Can you work these out from the model? Positions are in its coordinate system, mm. Round coordinates to 2 decimals unless told otherwise and drop trailing zeros. Write each question's results on one line, items separated by ' | '.
Autodesk Inventor part; units mm, degrees
ref_plane "YZ Plane" through (0, 0, 0) normal (1, 0, 0) x (0, 1, 0)
ref_plane "XZ Plane" through (0, 0, 0) normal (0, 1, 0) x (-1, 0, 0)
ref_plane "XY Plane" through (0, 0, 0) normal (0, 0, 1) x (1, 0, 0)
sketch "Sketch1" plane through (0, 0, 0) normal (0, 0, 1) x (1, 0, 0)
  line L0 (-90, -105) -> (90, -105)
  line L1 (90, -105) -> (90, 105)
  line L2 (-90, 105) -> (-90, -105)
  line L3 (42, 105) -> (42, 197)
  line L4 (42, 197) -> (-42, 197)
  line L5 (-42, 197) -> (-42, 105)
  line L6 (90, 105) -> (42, 105)
  line L7 (-42, 105) -> (-90, 105)
  point P0 (0, 0)
  dimension "d0" = 180
  dimension "d1" = 210
  dimension "d2" = 105
  dimension "d3" = 90
  dimension "d22" = 92
  dimension "d24" = 42
  dimension "d26" = 84
  dimension "d28" = 92
  dimension "d29" = 210
  dimension "d30" = 48
  dimension "d31" = 48
extrude "Extrusion1" add sketch "Sketch1" along normal blind 2
sketch "Sketch2" plane through (0, 0, 2) normal (0, 0, 1) x (1, 0, 0)
  line L0 (-90, -105) -> (90, -105)
  line L1 (-42, 105) -> (-90, 105)
  point P0 (0, 0)
  point P1 (-75, 80)
  point P2 (75, 80)
  point P3 (-75, -90)
  point P4 (75, -90)
  dimension "d6" = 170
  dimension "d8" = 150
  dimension "d9" = 75
  dimension "d10" = 150
  dimension "d11" = 15
  dimension "d12" = 15
  dimension "d13" = 170
  dimension "d14" = 75
  dimension "d27" = 25
hole "Hole1" at (-75, 80, 2) at (75, 80, 2) at (-75, -90, 2) at (75, -90, 2) direction (0, 0, -1) diameter 4.2 end through all
sketch "Sketch3" plane through (0, 0, 2) normal (0, 0, 1) x (1, 0, 0)
  line L0 (-90, 105) -> (-90, -105)
  line L1 (90, 105) -> (42, 105)
  line L2 (-39, 116) -> (39, 116)
  line L3 (39, 116) -> (39, 194)
  line L4 (39, 194) -> (-39, 194)
  line L5 (-39, 194) -> (-39, 116)
  point P0 (0, 0)
  dimension "d46" = 78
  dimension "d47" = 39
  dimension "d48" = 78
  dimension "d49" = 11
extrude "Extrusion2" cut sketch "Sketch3" against normal blind 10
chamfer "Chamfer1" distance 16.5 angle 45 4 edges at (-39, 116, 1) (39, 116, 1) (-39, 194, 1) (39, 194, 1)
sketch "Sketch4" plane through (0, 0, 2) normal (0, 0, 1) x (1, 0, 0)
  line L0 (-35.75, 190.9) -> (35.75, 190.9) construction
  line L1 (35.75, 190.9) -> (35.75, 119.4) construction
  line L2 (35.75, 119.4) -> (-35.75, 119.4) construction
  line L3 (-35.75, 119.4) -> (-35.75, 190.9) construction
  line L4 (90, 105) -> (42, 105) construction
  point P0 (0, 0)
  dimension "d53" = 71.5
  dimension "d54" = 35.75
  dimension "d55" = 71.5
  dimension "d56" = 14.4
hole "Hole2" at (-35.75, 190.9, 2) at (35.75, 190.9, 2) at (-35.75, 119.4, 2) at (35.75, 119.4, 2) direction (0, 0, -1) diameter 4.2 end through all
sketch "Sketch5" plane through (0, 0, 2) normal (0, 0, 1) x (1, 0, 0)
  line L0 (-42, 197) -> (-42, 105)
  line L1 (-42, 105) -> (-39, 105)
  line L2 (-39, 105) -> (-39, 107)
  line L3 (-39, 107) -> (-42, 107)
  line L4 (-42, 107) -> (-42, 105)
  line L5 (90, 105) -> (42, 105)
  line L6 (42, 105) -> (39, 105)
  line L7 (39, 105) -> (39, 107)
  line L8 (39, 107) -> (42, 107)
  line L9 (42, 107) -> (42, 105)
  line L10 (-20, 105) -> (20, 105)
  line L11 (20, 105) -> (20, 107)
  line L12 (20, 107) -> (-20, 107)
  line L13 (-20, 107) -> (-20, 105)
  point P0 (0, 0)
  dimension "d64" = 2
  dimension "d65" = 2
  dimension "d66" = 2
  dimension "d67" = 3
  dimension "d68" = 3
  dimension "d69" = 40
  dimension "d70" = 20
extrude "Extrusion3" cut sketch "Sketch5" against normal blind 10
fillet "Fillet1" radius 1 8 edges at (-39, 105, 1) (-39, 107, 1) (-20, 107, 1) (-20, 105, 1) (20, 105, 1) (20, 107, 1) (39, 107, 1) (39, 105, 1)
equation "\"d28\" = d22"
equation "\"d20\" = Thickness"
equation "\"d48\" = d46"
equation "\"d55\" = d53"
equation "\"d62\" = Thickness"
equation "\"BendRadius\" = Thickness"
equation "\"BendReliefWidth\" = Thickness"
equation "\"BendReliefDepth\" = 0.5 * Thickness"
equation "\"CornerReliefSize\" = 4 * Thickness"
equation "\"MinimumRemnant\" = 2 * Thickness"
equation "\"TransitionRadius\" = BendRadius"
equation "\"JacobiRadiusSize\" = BendRadius"
equation "\"GapSize\" = Thickness"
properties part number "XGEN_hotbed-pcb-org"
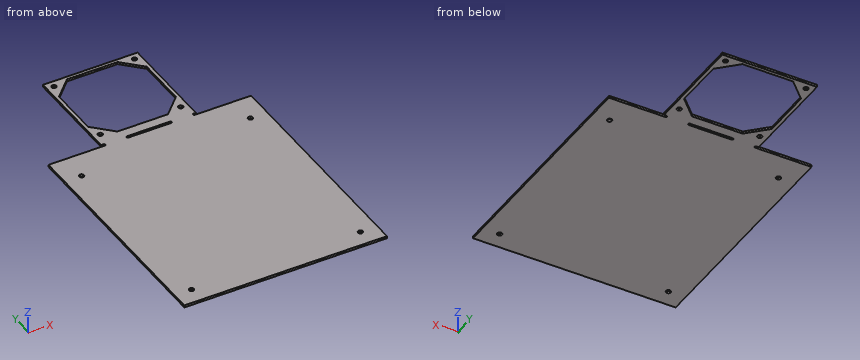
1. Will this pin go through, and if not, where does the flat tip stop? pin 1 (5.5 mm diameter, centred on x = 35.75, y = 190.9, fed in from -Z).
Final values:
pin 1: z = 0
2. Please list where these lines run through material, in increasing order: line 1 (X direction, y = -90.5, z = 1.2); line 2 (Y direction, x = -75, z = 1.65); line 3 (Y direction, x = 14.5, z = 1.4). Write a range as from..to.
Final values:
line 1: -90..-77.04, -72.96..72.96, 77.04..90 | line 2: -105..-92.1, -87.9..77.9, 82.1..105 | line 3: -105..105, 107..116, 194..197
3. If we section it at A-A (z = 0.3): State how many separate pieces and enclosed holes the cut face has, then the cut area to 3 significant figures.
Final values:
separate pieces: 1 | enclosed holes: 10 | area: 39,800 mm2
